Read the model definition and answer for the solid it produces. Units are mm, in the model's axes. A direction names the side the tool comes from. Round coordinates to 2 decimals unless told otherwise and drop trailing zeros. Order: outer loops, then holes, each group sorted by start corner. A loop starts at its lowest first (then second) coordinate and runs counter-clockwise, first axis right, second up. Notation, with made-up numbers: M 45.5,-4.5 L 58.5,-4.5 A16 cw 58.5,21.5 Z; hole C 0.5,10.5 d5. An arc over 180 degrees is marked long. Answer as CSV lines item,"result".
```python
from build123d import *

# Parameters (mm, degrees)
EXTRUDE_1_DEPTH     = 3
FILLET_1_R          = 2
SKETCH_2_R          = 1.5
CUT_EXTRUDE_1_DEPTH = 10
FILLET_3_R          = 1
SKETCH_3_W          = 76.2
SKETCH_3_H          = 3
EXTRUDE_2_DEPTH     = 3
FILLET_4_R          = 5


# Read off the part's stored shape, not the designer's step: 凸台-拉伸1
with BuildPart() as part:
    # 凸台-拉伸1 outline → 凸台-拉伸1 (new body)
    with BuildSketch(Plane.XY):
        with BuildLine():
            Line((76.2, -17), (76.2, -6))
            Line((76.2, -6), (73.2, -6))
            ThreePointArc((73.2, -6), (72.2, -5), (73.2, -4))
            Line((73.2, -4), (73.2, 0))
            Line((73.2, 0), (61.2, 0))
            Line((61.2, 0), (61.2, -6))
            Line((61.2, -6), (15, -6))
            Line((15, -6), (15, 0))
            Line((15, 0), (3, 0))
            Line((3, 0), (3, -4))
            ThreePointArc((3, -4), (4, -5), (3, -6))
            Line((3, -6), (0, -6))
            Line((0, -6), (0, -17))
            Line((0, -17), (76.2, -17))
        make_face()
        with BuildLine():
            Line((12, -10), (12, -13.5))
            ThreePointArc((12, -13.5), (10, -15.5), (8, -13.5))
            Line((8, -13.5), (8, -10))
            ThreePointArc((8, -10), (10, -8), (12, -10))
        make_face(mode=Mode.SUBTRACT)
        with BuildLine():
            Line((26.1, -13.5), (26.1, -10))
            ThreePointArc((26.1, -10), (28.1, -8), (30.1, -10))
            Line((30.1, -10), (30.1, -13.5))
            ThreePointArc((30.1, -13.5), (28.1, -15.5), (26.1, -13.5))
        make_face(mode=Mode.SUBTRACT)
        with BuildLine():
            Line((46.1, -13.5), (46.1, -10))
            ThreePointArc((46.1, -10), (48.1, -8), (50.1, -10))
            Line((50.1, -10), (50.1, -13.5))
            ThreePointArc((50.1, -13.5), (48.1, -15.5), (46.1, -13.5))
        make_face(mode=Mode.SUBTRACT)
        with BuildLine():
            Line((68.2, -10), (68.2, -13.5))
            ThreePointArc((68.2, -13.5), (66.2, -15.5), (64.2, -13.5))
            Line((64.2, -13.5), (64.2, -10))
            ThreePointArc((64.2, -10), (66.2, -8), (68.2, -10))
        make_face(mode=Mode.SUBTRACT)
    extrude(amount=EXTRUDE_1_DEPTH)

    # 圆角1
    fillet_1_edges = [part.edges().sort_by_distance(p)[0] for p in [
        (15, -6, 1.5),
        (61.2, -6, 1.5),
    ]]
    fillet(fillet_1_edges, radius=FILLET_1_R)

    # 草图2 → 切除-拉伸1 (cut)
    with BuildSketch(Plane.XY.offset(3)):
        with Locations((12, -3)):
            Circle(SKETCH_2_R)
        with Locations((64.2, -3)):
            Circle(SKETCH_2_R)
    extrude(amount=-CUT_EXTRUDE_1_DEPTH, mode=Mode.SUBTRACT)

    # 圆角3
    fillet_3_edges = [part.edges().sort_by_distance(p)[0] for p in [
        (15, 0, 1.5),
        (61.2, 0, 1.5),
    ]]
    fillet(fillet_3_edges, radius=FILLET_3_R)

    # 草图3 → 凸台-拉伸2 (add)
    with BuildSketch(Plane.XZ.offset(17)):
        with Locations((38.1, 1.5)):
            Rectangle(SKETCH_3_W, SKETCH_3_H)
    extrude(amount=EXTRUDE_2_DEPTH)

    # 圆角4
    fillet_4_edges = [part.edges().sort_by_distance(p)[0] for p in [
        (0, -20, 1.5),
        (76.2, -20, 1.5),
    ]]
    fillet(fillet_4_edges, radius=FILLET_4_R)


solid = part.part
```
Item 1: Flat-ended cylindrical pins translate along their axes: pin 1 (1.5 mm diameter, centred on x = 37.5, z = 1.5, fed in from +Y); pin 2 (1 mm diameter, centred on y = -17, z = 0.5, fed in from -X); pin 3 (1.5 mm diameter, centred on y = -2, z = 2, fed in from +X). Find the tip coordinate at first contact, or state that the pin passes through.
Ans:
pin 1,"y = -6"
pin 2,"x = 0.23"
pin 3,"x = 73.2"
Item 2: A cutting plane is placed at B-B, the plane y = -12. Determine the outline of the cut face in (x, z), and give its area (3 significant figures).
Ans:
outline,"M 0,0 L 8,0 L 8,3 L 0,3 Z; M 12,0 L 26.1,0 L 26.1,3 L 12,3 Z; M 30.1,0 L 46.1,0 L 46.1,3 L 30.1,3 Z; M 50.1,0 L 64.2,0 L 64.2,3 L 50.1,3 Z; M 68.2,0 L 76.2,0 L 76.2,3 L 68.2,3 Z"
area,"181 mm2"
Item 3: A cutting plane is placed at A-A, the plane x = 48.1. Determine the outline of the cut face in (y, z), and give its area (3 significant figures).
Ans:
outline,"M -20,0 L -15.5,0 L -15.5,3 L -20,3 Z; M -8,0 L -6,0 L -6,3 L -8,3 Z"
area,"19.5 mm2"
Item 4: A cutting plane is placed at C-C, the plane z = 1.8. Give the number of separate pieces and of enclosed holes in the cut face, and give its area (3 significant figures).
Ans:
separate pieces,"1"
enclosed holes,"6"
area,"1,080 mm2"
Item 5: A tool of negligible diameter and unlimited length cuts with its end or side. For faces 1 (the face through (73.2, -2, 1)), 2 (the face through (48.1, -8, 1.5)), 3 (the face through (61.2, -2, 1)), from which of +Z, -Z, +X, -X, +Y, -Y can it reach the whole face along a straight path? Write none if from no direction.
Ans:
face 1,"+Z, -Z, +X, +Y"
face 2,"+Z, -Z"
face 3,"+Z, -Z, +Y"
Item 6: A cutting plane is placed at D-D, the plane x = 37. Determine the outline of the cut face in (y, z), and give its area (3 significant figures).
Ans:
outline,"M -20,0 L -6,0 L -6,3 L -20,3 Z"
area,"42.0 mm2"
Item 7: Find the intervals of material crossed by probe 1 along X at (y, z) = (-12.5, 2.5); probe 2 along X at (y, z) = (-2.75, 1.1); probe 3 along X at (y, z) = (-5, 1.6), in increasing order. Write a range as [from, to].
Ans:
probe 1,"[0, 8], [12, 26.1], [30.1, 46.1], [50.1, 64.2], [68.2, 76.2]"
probe 2,"[3, 10.52], [13.48, 15], [61.2, 62.72], [65.68, 73.2]"
probe 3,"[4, 15.27], [60.93, 72.2]"
